from build123d import *

# Parameters (mm, degrees)
SKETCH1_R           = 4.7625
BOSS_EXTRUDE1_DEPTH = 2.778125
SKETCH5_OUTSIDE_W   = 43.504
SKETCH5_OUTSIDE_H   = 45.714
SKETCH5_OUTSIDE_R   = 7.14375
CUT_EXTRUDE2_DEPTH  = 6.55625
CUT_EXTRUDE2_TAPER  = 60


with BuildPart() as part:
    # Sketch1 → Boss-Extrude1 (new body, symmetric)
    with BuildSketch(Plane(origin=(0, 0, 0), x_dir=(1, 0, 0), z_dir=(0, 1, 0))):
        Polygon((-7.14375, 4.124445986), (-7.14375, -4.124445986), (0, -8.248891971), (7.14375, -4.124445986), (7.14375, 4.124445986), (0, 8.248891971), align=None)
        Circle(SKETCH1_R, mode=Mode.SUBTRACT)
    extrude(amount=BOSS_EXTRUDE1_DEPTH, both=True)

    # Sketch5 outside → Cut-Extrude2 (cut, through all)
    with BuildSketch(Plane(origin=(0, 2.778125, 0), x_dir=(1, 0, 0), z_dir=(0, 1, 0))):
        Rectangle(SKETCH5_OUTSIDE_W, SKETCH5_OUTSIDE_H)
        Circle(SKETCH5_OUTSIDE_R, mode=Mode.SUBTRACT)
    extrude(amount=-CUT_EXTRUDE2_DEPTH, taper=CUT_EXTRUDE2_TAPER, mode=Mode.SUBTRACT)


solid = part.part
Input: part model. Units: mm. Frame: model coordinates. Give positions to 0.01 mm unless a question says otherwise; leave off trailing zeros. Write each loop counter-clockwise with the first axis right and the second up, starting at its lowest first coordinate (ties: lowest second). Pieces come first, ordered by that corner, then holes.
Q1. First-contact query: P1, Ø5.5, axis at x = 0, z = 0, coming from the +Y side; P2, Ø3, axis at x = -5, y = 1.5, coming from the -Z side. Flat tips, straight axial feed; report the tip coordinate or a pass-through.
Q2. Pull-direction query (Z, two-part tool) for faces 1 (the face through (6.428, 2.623, 3.69)), 2 (the face through (-3.78, -0.04, 2.9)), 3 (the face through (-6.428, 2.623, -3.69)); classes: pulls with the +Z half, pulls with the -Z half, needs draft (parallel to the pull), parting line crosses it, or undercut.
Q3. Section A-A, the plane y = -1.5. Output: boundary loops of the cut face in (x, z) (1 decimal).
Q4. Material intervals for probe 1 along X at (y, z) = (0.9, 0); probe 2 along X at (y, z) = (-0.05, 1); probe 3 along X at (y, z) = (2.15, -5.5), sorted ascending.
Filled in:
1. P1: passes through
1. P2: stops at z = -6.23
2. face 1: pulls with the +Z half
2. face 2: undercut
2. face 3: pulls with the -Z half
3. outline: (-7.1, -4.1) - (0, -8.2) - (7.1, -4.1) - (7.1, 4.1) - (0, 8.2) - (-7.1, 4.1) - close; hole circle Ø9.5 at (0, 0)
4. probe 1: x = -7.14 to -4.76, 4.76 to 7.14
4. probe 2: x = -7.14 to -4.66, 4.66 to 7.14
4. probe 3: x = -4.76 to 4.76
